Here's how the part is built. I have some questions about the finished solid (model axes, mm). Coordinates: 2 decimals unless noted, no trailing zeros. Loops run counter-clockwise (first coordinate to the right, second up) from the corner with the lowest first, then second, coordinate; pieces in that order, holes last. Notation, with made-up numbers: (-8.75, -25.5) -> (27.25, -25.5) arc R12 cw to (27.25, -21.5) -> close; hole circle Ø9 at (11.5, -31.5). An arc over 180 degrees is marked (long way). Use CSV: the item, a comma, the result in double quotes. Start each with the question number.
from build123d import *

# Parameters (mm, degrees)
F0_W     = 508
F0_H     = 508
F0_R     = 127
F1_DEPTH = 25.4
F2_SIZE  = 50.8


with BuildPart() as f1:
    # F0 (on Top) → F1 (new body)
    with BuildSketch(Plane.XY):
        Rectangle(F0_W, F0_H)
        Circle(F0_R, mode=Mode.SUBTRACT)
    extrude(amount=F1_DEPTH)

    # F2
    f2_edges = [f1.edges().sort_by_distance(p)[0] for p in [
        (-254, -254, 12.7),
        (254, -254, 12.7),
        (254, 254, 12.7),
        (-254, 254, 12.7),
    ]]
    chamfer(f2_edges, length=F2_SIZE)


solid = f1.part
1) Thinking about a two-plate mould opening in Y: for faces 1 (the face through (229, -228.2, 12.5)), 2 (the face through (-27.53, -123.98, 12.52)), 3 (the face through (229, 228.2, 12.5)), which applies, pulls with the +Y half, pulls with the -Y half, needs draft (parallel to the pull), parting line crosses it, or undercut?
2) For P1, Ø1.5, axis at x = 116.5, y = -183, coming from the -Z side, with a flat end and sliding along its axis, tell me the tip position at first contact or that it passes through.
3) I want a section at B-B, the plane z = 8. Please give me the cut outline in (x, y), plus the area to 3 significant figures.
4) I want a section at A-A, the plane y = 0. Please give me the cut outline in (x, z).
5) Please list where these lines run through material, in increasing order: L1, parallel to Y at x = 0, z = 11.75; L2, parallel to Y at x = 45, z = 8.25; L3, parallel to X at y = 47, z = 2.5. Write a range as [from, to].
Return value:
1,face 1,"pulls with the -Y half"
1,face 2,"undercut"
1,face 3,"pulls with the +Y half"
2,P1,"stops at z = 0"
3,outline,"(-254, -203.2) -> (-203.2, -254) -> (203.2, -254) -> (254, -203.2) -> (254, 203.2) -> (203.2, 254) -> (-203.2, 254) -> (-254, 203.2) -> close; hole circle Ø254 at (0, 0)"
3,area,"202,000 mm²"
4,outline,"(-254, 0) -> (-127, 0) -> (-127, 25.4) -> (-254, 25.4) -> close; (127, 0) -> (254, 0) -> (254, 25.4) -> (127, 25.4) -> close"
5,L1,"y = [-254, -127], [127, 254]"
5,L2,"y = [-254, -118.76], [118.76, 254]"
5,L3,"x = [-254, -117.98], [117.98, 254]"
